```python
from build123d import *

# Parameters (mm, degrees)
SKETCH1_W               = 190
SKETCH1_H               = 190
BASE_DEPTH              = 4
SKETCH1_5_R             = 2.1
CUT_EXTRUDE2_DEPTH      = 4
MIRROR2_COPY_1_SKETCH_R = 2.1
MIRROR2_COPY_1_DEPTH    = 4
SKETCH2_R               = 2.55
SKETCH2_R_2             = 3.6
HOLES_DEPTH             = 5
CUT_EXTRUDE4_DEPTH      = 4
CUT_EXTRUDE5_DEPTH      = 4
CUT_EXTRUDE6_DEPTH      = 4
FILLET1_R               = 8
CUT_EXTRUDE7_DEPTH      = 4


with BuildPart() as part:
    # Sketch1 → base (new body)
    with BuildSketch(Plane(origin=(0, 0, 0), x_dir=(1, 0, 0), z_dir=(0, 1, 0))):
        Rectangle(SKETCH1_W, SKETCH1_H)
    extrude(amount=-BASE_DEPTH)

    # Sketch1_5 → Cut-Extrude2 (cut)
    with BuildSketch(Plane(origin=(0, 0, 0), x_dir=(1, 0, 0), z_dir=(0, 1, 0))):
        with Locations((-85, 85)):
            Circle(SKETCH1_5_R)
    cut_extrude2 = extrude(amount=-CUT_EXTRUDE2_DEPTH, mode=Mode.SUBTRACT)

    # Mirror1: Cut-Extrude2 across plane
    add(cut_extrude2.mirror(Plane(origin=(0, 0, 0), x_dir=(0, 0, 1), z_dir=(1, 0, 0))), mode=Mode.SUBTRACT)

    # Mirror2: Cut-Extrude2 across plane
    add(cut_extrude2.mirror(Plane.XY), mode=Mode.SUBTRACT)

    # Mirror2 copy 1 sketch → Mirror2 copy 1 (cut)
    with BuildSketch(Plane(origin=(0, 0, 0), x_dir=(-1, 0, 0), z_dir=(0, 1, 0))):
        with Locations((-85, 85)):
            Circle(MIRROR2_COPY_1_SKETCH_R)
    extrude(amount=-MIRROR2_COPY_1_DEPTH, mode=Mode.SUBTRACT)

    # Sketch2 → holes (cut, through all)
    with BuildSketch(Plane(origin=(0, 0, 0), x_dir=(1, 0, 0), z_dir=(0, 1, 0))):
        with Locations((-26.5, 27)):
            Circle(SKETCH2_R)
        with Locations((-26.5, -13)):
            Circle(SKETCH2_R)
        with Locations((26.5, -32)):
            Circle(SKETCH2_R_2)
        with Locations((26.5, 8)):
            Circle(SKETCH2_R_2)
    extrude(amount=-HOLES_DEPTH, mode=Mode.SUBTRACT)

    # Sketch3 → Cut-Extrude4 (cut)
    with BuildSketch(Plane(origin=(0, 0, 0), x_dir=(1, 0, 0), z_dir=(0, 1, 0))):
        Polygon((-45.366645318, 45.366645318), (0, 45.366645318), (18.398695046, 45.366645318), (30.496467131, 95), (-59.732749669, 95), align=None)
        Polygon((-51.667568279, -95), (50.911457524, -95), (30.496467131, -44.610534563), (-29.740356375, -44.610534563), align=None)
    extrude(amount=-CUT_EXTRUDE4_DEPTH, mode=Mode.SUBTRACT)

    # Sketch5 → Cut-Extrude5 (cut)
    with BuildSketch(Plane(origin=(0, 0, 0), x_dir=(1, 0, 0), z_dir=(0, 1, 0))):
        with BuildLine():
            Line((-95, 75.359038612), (-95, -75.107001693))
            ThreePointArc((-95, -75.107001693), (-73.504234295, 0.126018459), (-95, 75.359038612))
        make_face()
    extrude(amount=-CUT_EXTRUDE5_DEPTH, mode=Mode.SUBTRACT)

    # Sketch5_3 → Cut-Extrude6 (cut)
    with BuildSketch(Plane(origin=(0, 0, 0), x_dir=(1, 0, 0), z_dir=(0, 1, 0))):
        with BuildLine():
            Line((-95, 75.359038612), (-95, -75.107001693))
            ThreePointArc((-95, -75.107001693), (-73.504234295, 0.126018459), (-95, 75.359038612))
        make_face()
        with BuildLine():
            Line((95, -75.107001693), (95, 77.879407796))
            ThreePointArc((95, 77.879407796), (72.661894517, 1.386203051), (95, -75.107001693))
        make_face()
    extrude(amount=-CUT_EXTRUDE6_DEPTH, mode=Mode.SUBTRACT)

    # Fillet1
    fillet1_edges = [part.edges().sort_by_distance(p)[0] for p in [
        (95, -2, -77.879407796),
        (18.398695046, -2, -45.366645318),
        (-45.366645318, -2, -45.366645318),
        (-59.732749669, -2, -95),
        (30.496467131, -2, -95),
        (30.496467131, -2, 44.610534563),
        (50.911457524, -2, 95),
        (-51.667568279, -2, 95),
        (-29.740356375, -2, 44.610534563),
        (-95, -2, -95),
        (-95, -2, 95),
        (95, -2, 95),
        (95, -2, -95),
        (-95, -2, -75.359038612),
        (-95, -2, 75.107001693),
        (95, -2, 75.107001693),
    ]]
    fillet(fillet1_edges, radius=FILLET1_R)

    # Sketch7 → Cut-Extrude7 (cut)
    with BuildSketch(Plane(origin=(0, 0, 0), x_dir=(1, 0, 0), z_dir=(0, 1, 0))):
        Polygon((5, 45.366645318), (5, 40.366645318), (-3.5, 40.366645318), (-3.5, 37.866645318), (7.5, 37.866645318), (7.5, 45.366645318), align=None)
    cut_extrude7 = extrude(amount=-CUT_EXTRUDE7_DEPTH, mode=Mode.SUBTRACT)

    # Mirror3: Cut-Extrude7 across plane
    add(cut_extrude7.mirror(Plane.XY), mode=Mode.SUBTRACT)


solid = part.part
```
Geometry check sheet. Reference: the model listing, model coordinates, mm. A direction names the side the tool comes from. Round coordinates to 2 decimals unless told otherwise and drop trailing zeros. Order: outer loops, then holes, each group sorted by start corner. A loop starts at its lowest first (then second) coordinate and runs counter-clockwise, first axis right, second up. Notation, with made-up numbers: (58, 27.25) - (92, 27.25) arc R17 cw to (92, 55.25) - close; hole circle Ø11 at (-3, 11). An arc over 180 degrees is marked (long way). Use a Markdown table: item, result. Add a question column.
1) Thickness scan on line 1 along Z through (x, y) = (-2.5, -1.6); line 2 along X through (y, z) = (-3.65, -86.5); line 3 along X through (y, z) = (-2, 38). Record the ranges inside material, lowest first.
2) Section check C-C (y = -1.65). Count the separate pieces of the cut face and the enclosed holes in it, then the cut area to 3 significant figures.
3) Section check D-D (x = -11). Record the cut outline in (y, z).
4) Mould release check, pull along Z, two halves, no side actions. Record for faces 1 (the cylindrical face through (87.1, -1.97, 85.09)), 2 (the flat face through (-52.627, -1.972, -70.45)), 3 (the cylindrical face through (-92.719, -2.028, 92.594)): released by +Z, released by -Z, zero draft, split by the parting line, or undercut.
5) Section check B-B (x = 80.5). Record the cut outline in (y, z).
6) Set-up check for faces 4 (the flat face through (40.82, -1.97, 70.09)), 5 (the cylindrical face through (-92.719, -2.028, -92.594)), 6 (the flat face through (24.384, -1.972, -69.921)): record each of +Z, -Z, +X, -X, +Y, -Y from which the full face is reachable in a straight line by a thin tool's end or side.
7) Gauge pin test, flat ends, axial feed: P1, Ø0.8, axis at y = -2.5, z = -39, coming from the +X side; P2, Ø1, axis at y = -3, z = -3, coming from the +X side; P3, Ø2, axis at x = -7, y = -1.5, coming from the -Z side; P4, Ø3.5, axis at x = 85, z = 85, coming from the -Y side. Record the tip position at first contact, or that the pin passes through.
8) Section check A-A (z = -8). Record the cut outline in (x, y).
Established:
| question | item | result |
|---|---|---|
| 1 | line 1 | -45.37 to -40.37, -37.87 to 37.87, 40.37 to 44.61 |
| 1 | line 2 | -95 to -86.47, -83.53 to -57.27, 28.42 to 83.53, 86.47 to 95 |
| 1 | line 3 | -78.7 to -3.5, 7.5 to 78.23 |
| 2 | separate pieces | 1 |
| 2 | enclosed holes | 8 |
| 2 | area | 23,400 mm2 |
| 3 | outline | (-4, -45.37) - (0, -45.37) - (0, 44.61) - (-4, 44.61) - close |
| 4 | face 1 | undercut |
| 4 | face 2 | released by -Z |
| 4 | face 3 | released by +Z |
| 5 | outline | (-4, -95) - (0, -95) - (0, -47.93) - (-4, -47.93) - close; (-4, 45.16) - (0, 45.16) - (0, 95) - (-4, 95) - close |
| 6 | face 4 | +Z, +Y, -Y |
| 6 | face 5 | -Z, -X, +Y, -Y |
| 6 | face 6 | -Z, +Y, -Y |
| 7 | P1 | x = 77.84 |
| 7 | P2 | x = 72.68 |
| 7 | P3 | z = -45.37 |
| 7 | P4 | through |
| 8 | outline | (-73.72, -4) - (22.9, -4) - (22.9, 0) - (-73.72, 0) - close; (30.1, -4) - (72.82, -4) - (72.82, 0) - (30.1, 0) - close |
